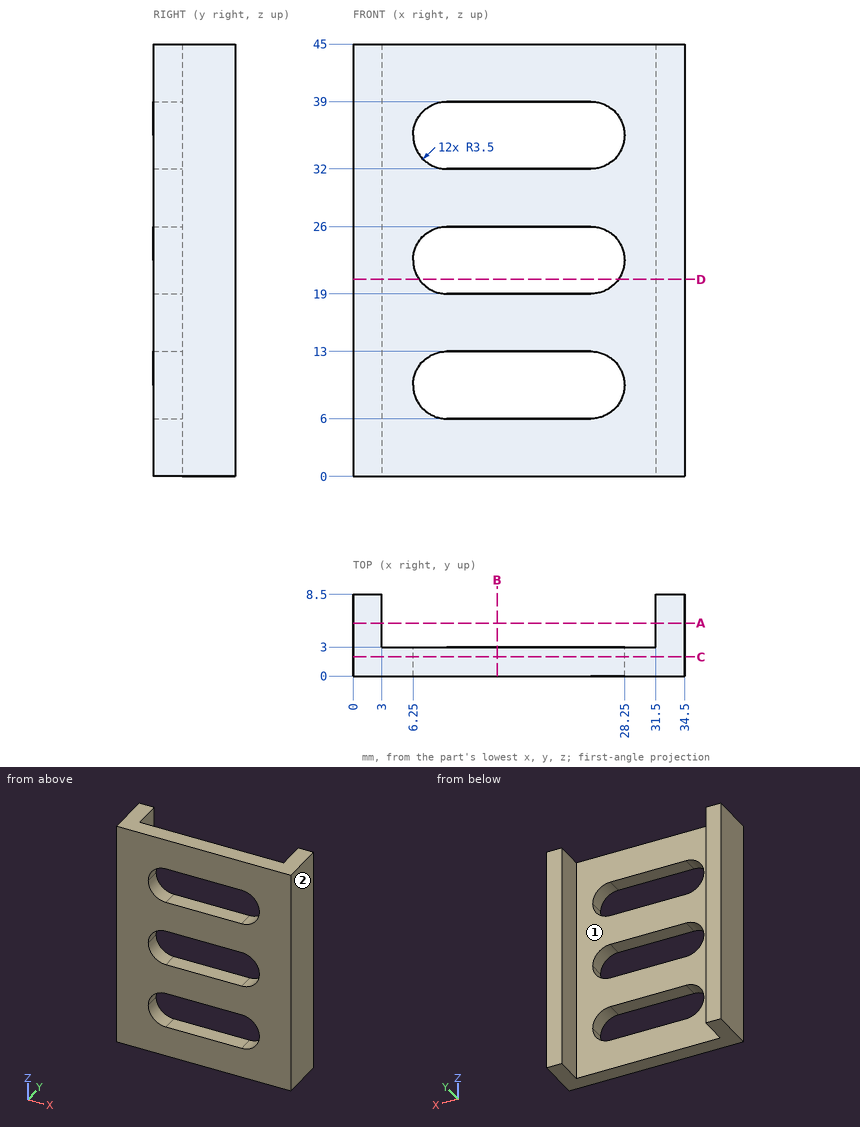
Could you check a few things on this drawing? It's one solid part, dimensions in mm from its lowest x, y, z. A direction names the side the tool comes from. Round coordinates to 2 decimals unless told otherwise and drop trailing zeros. Order: outer loops, then holes, each group sorted by start corner. A loop starts at its lowest first (then second) coordinate and runs counter-clockwise, first axis right, second up. Notation, with made-up numbers: M -4,49.25 L 49,49.25 A18 cw 49,53.25 Z; hole C -5.5,-5 d6. An arc over 180 degrees is marked long. Use a Markdown table: item, result.
1) I'm going to push flat-ended pins straight in: P1, Ø2.5, axis at x = 13.5, y = 1, coming from the -Z side; P2, Ø4, axis at x = 23.5, z = 13.5, coming from the +Y side. Where does each tip first touch, or does it pass through?
Geometry says:
| item | result |
|---|---|
| P1 | stops at z = 0 |
| P2 | stops at y = 3 |
2) Imagine slicing it at A-A (y = 5.5). List the corners of the cut face in (x, z) for me.
Geometry says:
| item | result |
|---|---|
| outline | M 0,0 L 3,0 L 3,45 L 0,45 Z; M 31.5,0 L 34.5,0 L 34.5,45 L 31.5,45 Z |
3) If I drill on line 1 along Z through (x, y) = (23, 0.5); line 2 along X through (y, z) = (5, 25); line 3 along Z through (x, y) = (27, 0.5), over which ranges is the centre line in solid material (lowest first)?
Geometry says:
| item | result |
|---|---|
| line 1 | z = 0 to 6, 13 to 19, 26 to 32, 39 to 45 |
| line 2 | x = 0 to 3, 31.5 to 34.5 |
| line 3 | z = 0 to 6.82, 12.18 to 19.82, 25.18 to 32.82, 38.18 to 45 |
4) Imagine slicing it at B-B (x = 15). List the corners of the cut face in (y, z) for me, then the cut area to 3 significant figures.
Geometry says:
| item | result |
|---|---|
| outline | M 0,0 L 3,0 L 3,6 L 0,6 Z; M 0,13 L 3,13 L 3,19 L 0,19 Z; M 0,26 L 3,26 L 3,32 L 0,32 Z; M 0,39 L 3,39 L 3,45 L 0,45 Z |
| area | 72.0 mm² |
5) Imagine slicing it at D-D (z = 20.5). List the corners of the cut face in (x, y) for me.
Geometry says:
| item | result |
|---|---|
| outline | M 0,0 L 6.88,0 L 6.88,3 L 3,3 L 3,8.5 L 0,8.5 Z; M 27.62,0 L 34.5,0 L 34.5,8.5 L 31.5,8.5 L 31.5,3 L 27.62,3 Z |
6) Imagine slicing it at C-C (y = 2). Give the number of separate pieces and of enclosed holes in the cut face, then the cut area to 3 significant figures.
Geometry says:
| item | result |
|---|---|
| separate pieces | 1 |
| enclosed holes | 3 |
| area | 1,120 mm² |
7) On a 3-axis mill with a long thin cutter (end or side, diameter ignored), from which of +Z, -Z, +X, -X, +Y, -Y can I reach the whole of each face in a straight line? I mean the marked faces 1 and 2. Say none if no direction works.
Geometry says:
| item | result |
|---|---|
| face 1 | +Z, -Z, +Y |
| face 2 | +Z, -Z, +X, +Y, -Y |
